```python
from build123d import *

# Parameters (mm, degrees)
SKETCH1_R              = 11.4
SKETCH1_R_2            = 1.8
SKETCH1_R_3            = 2.3
SKETCH1_R_4            = 4
BOSS_EXTRUDE1_DEPTH    = 7
CHAMFER2_SIZE          = 2
CUT_EXTRUDE2_DEPTH     = 196.146842147
SKETCH4_R              = 1.5
CUT_EXTRUDE3_DEPTH     = 196.146842147
SKETCH6_R              = 7.1
CUT_EXTRUDE4_DEPTH     = 5
SKETCH7_R              = 2.3
CUT_EXTRUDE5_DEPTH     = 10
CUT_EXTRUDE6_DEPTH     = 10
MOVE_START             = 6
MOVE_FACE2_OUTLINE_R   = 2.3
MOVE_FACE2_OUTLINE_R_2 = 1.5
MOVE_FACE2_OUTLINE_R_3 = 1.8
MOVE_FACE2_OUTLINE_R_4 = 11.4
MOVE_FACE2_OUTLINE_R_5 = 4
MOVE_FACE2_DEPTH       = 1


# Read off the part's stored shape, not the designer's step: Move Face2
with BuildPart() as part:
    # Sketch1 → Boss-Extrude1 (new body)
    with BuildSketch(Plane(origin=(0, 0, 0), x_dir=(0, 0, -1), z_dir=(1, 0, 0))):
        with BuildLine():
            Line((-168.7, 24), (-30, 24))
            ThreePointArc((-30, 24), (-25.757359313, 25.757359313), (-24, 30))
            Line((-24, 30), (-12, 30))
            Line((-12, 30), (0, 30))
            Line((0, 30), (0, 24))
            Line((0, 24), (0, 0))
            Line((0, 0), (0, -24))
            Line((0, -24), (0, -30))
            Line((0, -30), (-12, -30))
            Line((-12, -30), (-24, -30))
            ThreePointArc((-24, -30), (-25.757359313, -25.757359313), (-30, -24))
            Line((-30, -24), (-168.7, -24))
            ThreePointArc((-168.7, -24), (-192.7, 0), (-168.7, 24))
        make_face()
        with Locations((-68.3, 0)):
            Circle(SKETCH1_R, mode=Mode.SUBTRACT)
        with Locations((-83.8, 15.5)):
            Circle(SKETCH1_R_2, mode=Mode.SUBTRACT)
        with Locations((-52.8, 15.5)):
            Circle(SKETCH1_R_2, mode=Mode.SUBTRACT)
        with Locations((-83.8, -15.5)):
            Circle(SKETCH1_R_2, mode=Mode.SUBTRACT)
        with Locations((-52.8, -15.5)):
            Circle(SKETCH1_R_2, mode=Mode.SUBTRACT)
        with Locations((-12, 16.5)):
            Circle(SKETCH1_R_3, mode=Mode.SUBTRACT)
        with Locations((-12, 0)):
            Circle(SKETCH1_R_3, mode=Mode.SUBTRACT)
        with Locations((-12, -16.5)):
            Circle(SKETCH1_R_3, mode=Mode.SUBTRACT)
        with Locations((-168.7, 0)):
            Circle(SKETCH1_R_4, mode=Mode.SUBTRACT)
    extrude(amount=BOSS_EXTRUDE1_DEPTH)

    # Chamfer2
    chamfer2_edges = [part.edges().sort_by_distance(p)[0] for p in [
        (0, -25.757359313, 25.757359313),
        (0, -24, 99.35),
        (0, 0, 192.7),
        (0, 24, 99.35),
        (0, 25.757359313, 25.757359313),
    ]]
    chamfer(chamfer2_edges, length=CHAMFER2_SIZE)

    # Sketch3 → Cut-Extrude2 (cut, through all)
    with BuildSketch(Plane(origin=(7, 0, 0), x_dir=(0, 0, -1), z_dir=(1, 0, 0))):
        with BuildLine():
            Line((-114.233163347, 15.207239819), (-114.233163347, 9.807239819))
            ThreePointArc((-114.233163347, 9.807239819), (-116.933163347, 7.107239819), (-119.633163347, 9.807239819))
            Line((-119.633163347, 9.807239819), (-119.633163347, 15.207239819))
            ThreePointArc((-119.633163347, 15.207239819), (-116.933163347, 17.907239819), (-114.233163347, 15.207239819))
        make_face()
    extrude(amount=-CUT_EXTRUDE2_DEPTH, mode=Mode.SUBTRACT)

    # Sketch4 → Cut-Extrude3 (cut, through all)
    with BuildSketch(Plane.ZY):
        with Locations((108.35, -20.4)):
            Circle(SKETCH4_R)
        with Locations((168.7, -20.4)):
            Circle(SKETCH4_R)
        with Locations((168.7, 20.4)):
            Circle(SKETCH4_R)
        with Locations((183.124978336, 14.424978336)):
            Circle(SKETCH4_R)
        with Locations((189.1, 0)):
            Circle(SKETCH4_R)
        with Locations((183.124978336, -14.424978336)):
            Circle(SKETCH4_R)
        with Locations((108.35, 20.4)):
            Circle(SKETCH4_R)
        with Locations((48, -20.4)):
            Circle(SKETCH4_R)
        with Locations((48, 20.4)):
            Circle(SKETCH4_R)
    extrude(amount=-CUT_EXTRUDE3_DEPTH, mode=Mode.SUBTRACT)

    # Sketch6 → Cut-Extrude4 (cut)
    with BuildSketch(Plane.ZY):
        with Locations((168.7, 0)):
            Circle(SKETCH6_R)
    extrude(amount=-CUT_EXTRUDE4_DEPTH, mode=Mode.SUBTRACT)

    # Sketch7 → Cut-Extrude5 (cut)
    with BuildSketch(Plane(origin=(7, 0, 0), x_dir=(0, 0, -1), z_dir=(1, 0, 0))):
        with Locations((-129.6, 0)):
            Circle(SKETCH7_R)
    extrude(amount=-CUT_EXTRUDE5_DEPTH, mode=Mode.SUBTRACT)

    # Sketch8 → Cut-Extrude6 (cut)
    with BuildSketch(Plane(origin=(7, 0, 0), x_dir=(0, 0, -1), z_dir=(1, 0, 0))):
        with BuildLine():
            Line((-97.45, -5), (-100.45, -5))
            ThreePointArc((-100.45, -5), (-101.45, -4), (-100.45, -3))
            Line((-100.45, -3), (-97.45, -3))
            ThreePointArc((-97.45, -3), (-96.45, -4), (-97.45, -5))
        make_face()
        with BuildLine():
            Line((-97.45, 5), (-100.45, 5))
            ThreePointArc((-100.45, 5), (-101.45, 4), (-100.45, 3))
            Line((-100.45, 3), (-97.45, 3))
            ThreePointArc((-97.45, 3), (-96.45, 4), (-97.45, 5))
        make_face()
        with BuildLine():
            Line((-40.2, -5), (-43.2, -5))
            ThreePointArc((-43.2, -5), (-44.2, -4), (-43.2, -3))
            Line((-43.2, -3), (-40.2, -3))
            ThreePointArc((-40.2, -3), (-39.2, -4), (-40.2, -5))
        make_face()
        with BuildLine():
            Line((-40.2, 5), (-43.2, 5))
            ThreePointArc((-43.2, 5), (-44.2, 4), (-43.2, 3))
            Line((-43.2, 3), (-40.2, 3))
            ThreePointArc((-40.2, 3), (-39.2, 4), (-40.2, 5))
        make_face()
    extrude(amount=-CUT_EXTRUDE6_DEPTH, mode=Mode.SUBTRACT)

    # Move Face2 outline → Move Face2 (cut)
    with BuildSketch(Plane.YZ.offset(MOVE_START)):
        with BuildLine():
            Line((-30, 24), (-30, 0))
            Line((-30, 0), (30, 0))
            Line((30, 0), (30, 24))
            ThreePointArc((30, 24), (25.757359313, 25.757359313), (24, 30))
            Line((24, 30), (24, 168.7))
            ThreePointArc((24, 168.7), (0, 192.7), (-24, 168.7))
            Line((-24, 168.7), (-24, 30))
            ThreePointArc((-24, 30), (-25.757359313, 25.757359313), (-30, 24))
        make_face()
        with Locations((-16.5, 12)):
            Circle(MOVE_FACE2_OUTLINE_R, mode=Mode.SUBTRACT)
        with Locations((-20.4, 48)):
            Circle(MOVE_FACE2_OUTLINE_R_2, mode=Mode.SUBTRACT)
        with BuildLine():
            Line((-5, 40.2), (-5, 43.2))
            ThreePointArc((-5, 43.2), (-4, 44.2), (-3, 43.2))
            Line((-3, 43.2), (-3, 40.2))
            ThreePointArc((-3, 40.2), (-4, 39.2), (-5, 40.2))
        make_face(mode=Mode.SUBTRACT)
        with Locations((-15.5, 52.8)):
            Circle(MOVE_FACE2_OUTLINE_R_3, mode=Mode.SUBTRACT)
        with Locations((-15.5, 83.8)):
            Circle(MOVE_FACE2_OUTLINE_R_3, mode=Mode.SUBTRACT)
        with Locations((0, 12)):
            Circle(MOVE_FACE2_OUTLINE_R, mode=Mode.SUBTRACT)
        with BuildLine():
            ThreePointArc((5, 40.2), (4, 39.2), (3, 40.2))
            Line((3, 40.2), (3, 43.2))
            ThreePointArc((3, 43.2), (4, 44.2), (5, 43.2))
            Line((5, 43.2), (5, 40.2))
        make_face(mode=Mode.SUBTRACT)
        with Locations((16.5, 12)):
            Circle(MOVE_FACE2_OUTLINE_R, mode=Mode.SUBTRACT)
        with Locations((20.4, 48)):
            Circle(MOVE_FACE2_OUTLINE_R_2, mode=Mode.SUBTRACT)
        with Locations((0, 68.3)):
            Circle(MOVE_FACE2_OUTLINE_R_4, mode=Mode.SUBTRACT)
        with Locations((15.5, 52.8)):
            Circle(MOVE_FACE2_OUTLINE_R_3, mode=Mode.SUBTRACT)
        with Locations((15.5, 83.8)):
            Circle(MOVE_FACE2_OUTLINE_R_3, mode=Mode.SUBTRACT)
        with Locations((-20.4, 108.35)):
            Circle(MOVE_FACE2_OUTLINE_R_2, mode=Mode.SUBTRACT)
        with BuildLine():
            ThreePointArc((-3, 97.45), (-4, 96.45), (-5, 97.45))
            Line((-5, 97.45), (-5, 100.45))
            ThreePointArc((-5, 100.45), (-4, 101.45), (-3, 100.45))
            Line((-3, 100.45), (-3, 97.45))
        make_face(mode=Mode.SUBTRACT)
        with Locations((-20.4, 168.7)):
            Circle(MOVE_FACE2_OUTLINE_R_2, mode=Mode.SUBTRACT)
        with Locations((-14.424978336, 183.124978336)):
            Circle(MOVE_FACE2_OUTLINE_R_2, mode=Mode.SUBTRACT)
        with BuildLine():
            Line((3, 97.45), (3, 100.45))
            ThreePointArc((3, 100.45), (4, 101.45), (5, 100.45))
            Line((5, 100.45), (5, 97.45))
            ThreePointArc((5, 97.45), (4, 96.45), (3, 97.45))
        make_face(mode=Mode.SUBTRACT)
        with BuildLine():
            ThreePointArc((15.207239819, 119.633163347), (17.907239819, 116.933163347), (15.207239819, 114.233163347))
            Line((15.207239819, 114.233163347), (9.807239819, 114.233163347))
            ThreePointArc((9.807239819, 114.233163347), (7.107239819, 116.933163347), (9.807239819, 119.633163347))
            Line((9.807239819, 119.633163347), (15.207239819, 119.633163347))
        make_face(mode=Mode.SUBTRACT)
        with Locations((0, 129.6)):
            Circle(MOVE_FACE2_OUTLINE_R, mode=Mode.SUBTRACT)
        with Locations((20.4, 108.35)):
            Circle(MOVE_FACE2_OUTLINE_R_2, mode=Mode.SUBTRACT)
        with Locations((0, 168.7)):
            Circle(MOVE_FACE2_OUTLINE_R_5, mode=Mode.SUBTRACT)
        with Locations((0, 189.1)):
            Circle(MOVE_FACE2_OUTLINE_R_2, mode=Mode.SUBTRACT)
        with Locations((14.424978336, 183.124978336)):
            Circle(MOVE_FACE2_OUTLINE_R_2, mode=Mode.SUBTRACT)
        with Locations((20.4, 168.7)):
            Circle(MOVE_FACE2_OUTLINE_R_2, mode=Mode.SUBTRACT)
    extrude(amount=MOVE_FACE2_DEPTH, mode=Mode.SUBTRACT)


solid = part.part
```
Could you check a few things on this model? Use its own coordinates, in mm. A direction names the side the tool comes from. Coordinates: 2 decimals unless noted, no trailing zeros. Order: outer loops, then holes, each group sorted by start corner. A loop starts at its lowest first (then second) coordinate and runs counter-clockwise, first axis right, second up. Notation, with made-up numbers: M 80.25,54.5 L 88.25,54.5 A11 ccw 88.25,69.5 Z; hole C -27.75,51 d1. An arc over 180 degrees is marked long. Use one line per item in the form item = value. Start each with the question number.
1. On a 3-axis mill with a long thin cutter (end or side, diameter ignored), from which of +Z, -Z, +X, -X, +Y, -Y can I reach the whole of each face in a straight line? I mean faces 1 (the conical face through (1.43, 25.3, 25.41)), 2 (the cylindrical face through (2.465, 2.133, 175.472)), 3 (the conical face through (1.43, -25.41, 25.3)), 4 (the flat face through (3, 12, 119.633)), 5 (the flat face through (4, -24, 98)). Say none if no direction works.
2. For pin 1 (3 mm diameter, centred on x = 3, z = 70.5, fed in from +Y); pin 2 (1 mm diameter, centred on x = 3.5, z = 27.5, fed in from +Y); pin 3 (2.5 mm diameter, centred on x = 3, z = 99, fed in from -Y), each with a flat end and sliding along its axis, tell me the tip position at first contact or that it passes through.
3. Suppose I cut it at A-A on z = 83.8. Write out the boundary of the cut face in (x, y), then the cut area to 3 significant figures.
4. Suppose I cut it at B-B on z = 117.5. Write out the boundary of the cut face in (x, y), then the cut area to 3 significant figures.
5. We'd pull the mould along Y, two halves only. Please class faces 6 (the cylindrical face through (2.958, 15.1, 13.825)), 7 (the flat face through (4, 24, 100)), 8 (the flat face through (0, 0, 94)): +Y half, -Y half, draft (parallel to the pull), parting line (faces both ways), or undercut.
6. Please list where these lines run through material, in increasing order: line 1 (Y direction, x = 2.85, z = 48); line 2 (Y direction, x = 1.85, z = 12); line 3 (Y direction, x = 2.75, z = 98).
Geometry says:
q1.face_1 = +Z, -X, +Y
q1.face_2 = -X
q1.face_3 = +Z, -X, -Y
q1.face_4 = +X, -X
q1.face_5 = +Z, +X, -X, -Y
q2.pin_1 = 24
q2.pin_2 = 24.8
q2.pin_3 = -24
q3.outline = M 0,-22 L 2,-24 L 6,-24 L 6,-17.3 L 0,-17.3 Z; M 0,-13.7 L 6,-13.7 L 6,13.7 L 0,13.7 Z; M 0,17.3 L 6,17.3 L 6,24 L 2,24 L 0,22 Z
q3.area = 241 mm^2
q4.outline = M 0,-22 L 2,-24 L 6,-24 L 6,7.17 L 0,7.17 Z; M 0,17.85 L 6,17.85 L 6,24 L 2,24 L 0,22 Z
q4.area = 220 mm^2
q5.face_6 = undercut
q5.face_7 = +Y half
q5.face_8 = draft
q6.line_1 = -24 to -21.9, -18.9 to 18.9, 21.9 to 24
q6.line_2 = -30 to -18.8, -14.2 to -2.3, 2.3 to 14.2, 18.8 to 30
q6.line_3 = -24 to -5, -3 to 3, 5 to 24
